```python
from build123d import *

# Parameters (mm, degrees)
CROQUIS1_W              = 180
CROQUIS1_H              = 65
SALIENTE_EXTRUIR1_DEPTH = 3
REDONDEO1_R             = 20
CROQUIS2_R              = 1.75
CORTAR_EXTRUIR1_DEPTH   = 3
CROQUIS3_R              = 1.75
CROQUIS3_R_2            = 4
CORTAR_EXTRUIR2_DEPTH   = 3
CROQUIS4_R              = 7.5
CORTAR_EXTRUIR3_DEPTH   = 200


with BuildPart() as part:
    # Croquis1 → Saliente-Extruir1 (new body)
    with BuildSketch(Plane(origin=(0, 0, 0), x_dir=(1, 0, 0), z_dir=(0, 1, 0))):
        Rectangle(CROQUIS1_W, CROQUIS1_H)
    extrude(amount=SALIENTE_EXTRUIR1_DEPTH)

    # Redondeo1
    redondeo1_edges = [part.edges().sort_by_distance(p)[0] for p in [
        (90, 1.5, 32.5),
        (-90, 1.5, 32.5),
        (-90, 1.5, -32.5),
        (90, 1.5, -32.5),
    ]]
    fillet(redondeo1_edges, radius=REDONDEO1_R)

    # Croquis2 → Cortar-Extruir1 (cut)
    with BuildSketch(Plane(origin=(0, 3, 0), x_dir=(1, 0, 0), z_dir=(0, 1, 0))):
        with Locations(Location((-80, 22.5, 0), (0, 0, 270))):
            Circle(CROQUIS2_R)
        with Locations(Location((-80, -22.5, 0), (0, 0, 270))):
            Circle(CROQUIS2_R)
        with Locations(Location((80, -22.5, 0), (0, 0, 270))):
            Circle(CROQUIS2_R)
        with Locations(Location((80, 22.5, 0), (0, 0, 270))):
            Circle(CROQUIS2_R)
    extrude(amount=-CORTAR_EXTRUIR1_DEPTH, mode=Mode.SUBTRACT)

    # Croquis3 → Cortar-Extruir2 (cut)
    with BuildSketch(Plane.XZ):
        with Locations(Location((-67, 16, 0), (0, 0, 270))):
            Circle(CROQUIS3_R)
        with Locations(Location((-59, 0, 0), (0, 0, 270))):
            Circle(CROQUIS3_R)
        with Locations(Location((-67, -16, 0), (0, 0, 270))):
            Circle(CROQUIS3_R)
        with Locations(Location((-67, 0, 0), (0, 0, 270))):
            Circle(CROQUIS3_R_2)
        with Locations(Location((-75, 0, 0), (0, 0, 270))):
            Circle(CROQUIS3_R)
    extrude(amount=-CORTAR_EXTRUIR2_DEPTH, mode=Mode.SUBTRACT)

    # Croquis4 → Cortar-Extruir3 (cut)
    with BuildSketch(Plane.XZ):
        with Locations(Location((-35, -17.5, 0), (0, 0, 270))):
            Circle(CROQUIS4_R)
    extrude(amount=-CORTAR_EXTRUIR3_DEPTH, mode=Mode.SUBTRACT)


solid = part.part
```
The listing builds one solid part. Answer for the finished solid, in the listing's coordinates (mm). Give positions to 0.01 mm unless a question says otherwise; leave off trailing zeros. Write each loop counter-clockwise with the first axis right and the second up, starting at its lowest first coordinate (ties: lowest second). Pieces come first, ordered by that corner, then holes. Notation, with made-up numbers: M 3.5,63.25 L 58.5,63.25 A16 ccw 58.5,77.25 Z; hole C 32.25,85 d8. An arc over 180 degrees is marked long. Write each question's results on one line, items separated by ' | '.
Q1. For a pull along Z with two mould halves and no side action, classify faces 1 (the cylindrical face through (-84.297, 1.521, -26.486)), 2 (the cylindrical face through (-68.71, 1.48, 16.38)), 3 (the flat face through (-1, 0, 0)) as released by +Z, released by -Z, zero draft, split by the parting line, or undercut.
Output values:
face 1: released by -Z | face 2: undercut | face 3: zero draft
Q2. Consider L1, parallel to X at y = 1.05, z = 0; L2, parallel to X at y = 2.1, z = 22.5; L3, parallel to X at y = 2.8, z = -24. Determine where each line is inside the solid, lowest interval first. Write a range as from..to.
Output values:
L1: -90..-76.75, -73.25..-71, -63..-60.75, -57.25..90 | L2: -87.32..-81.75, -78.25..78.25, 81.75..87.32 | L3: -86.36..-80.9, -79.1..-38.74, -31.26..79.1, 80.9..86.36
Q3. Section B-B, the plane z = 16 is taken. Write down the section's boundary in (x, y), then the cut area to 3 significant figures.
Output values:
outline: M -89.69,0 L -68.75,0 L -68.75,3 L -89.69,3 Z; M -65.25,0 L 89.69,0 L 89.69,3 L -65.25,3 Z | area: 528 mm2
Q4. Section A-A, the plane x = -59 is taken. Write down the section's boundary in (y, z), then the cut area to 4 significant figures.
Output values:
outline: M 0,-32.5 L 3,-32.5 L 3,-1.75 L 0,-1.75 Z; M 0,1.75 L 3,1.75 L 3,32.5 L 0,32.5 Z | area: 184.5 mm2
Q5. Section C-C, the plane y = 1.4 is taken. Count the separate pieces of the cut face and the enclosed holes in it, then the cut area to 3 significant figures.
Output values:
separate pieces: 1 | enclosed holes: 10 | area: 11,100 mm2
Q6. Section D-D, the plane z = 0 is taken. Write down the section's boundary in (x, y).
Output values:
outline: M -90,0 L -76.75,0 L -76.75,3 L -90,3 Z; M -73.25,0 L -71,0 L -71,3 L -73.25,3 Z; M -63,0 L -60.75,0 L -60.75,3 L -63,3 Z; M -57.25,0 L 90,0 L 90,3 L -57.25,3 Z
Q7. Flat-ended cylindrical pins translate along their axes: P1, Ø9, axis at x = -35, z = -17.5, coming from the -Y side; P2, Ø1, axis at y = 1.5, z = 17.5, coming from the +X side. Find the tip coordinate at first contact, or state that the pin passes through.
Output values:
P1: through | P2: x = 89.49
